Geometry: final body of the model. Coordinates: model frame, mm. A direction names the side the tool comes from. Give positions to 0.01 mm unless a question says otherwise; leave off trailing zeros. Order: outer loops, then holes, each group sorted by start corner. A loop starts at its lowest first (then second) coordinate and runs counter-clockwise, first axis right, second up. Notation, with made-up numbers: (-15, 27) - (38, 27) arc R20 cw to (38, 54) - close; hole circle Ø4 at (18.5, 75.25). An arc over 180 degrees is marked (long way). Use one line per item in the form item = value.
from build123d import *

# Parameters (mm, degrees)
SKETCH1_R           = 1.5
BOSS_EXTRUDE1_DEPTH = 1.5


with BuildPart() as part:
    # Sketch1 → Boss-Extrude1 (new body)
    with BuildSketch(Plane(origin=(0, 0, 0), x_dir=(1, 0, 0), z_dir=(0, 1, 0))):
        with BuildLine():
            Line((6.755042478, -2), (69.244957522, -2))
            ThreePointArc((69.244957522, -2), (70.169022091, -2.617763592), (69.951379765, -3.707790657))
            Line((69.951379765, -3.707790657), (67.996333944, -5.65905667))
            ThreePointArc((67.996333944, -5.65905667), (67.993254266, -9.902722426), (72.236921016, -9.903748986))
            Line((72.236921016, -9.903748986), (74.292893219, -7.847776783))
            ThreePointArc((74.292893219, -7.847776783), (75.382683432, -7.631004031), (76, -8.554883564))
            Line((76, -8.554883564), (76, -49.445116436))
            ThreePointArc((76, -49.445116436), (75.382683432, -50.368995969), (74.292893219, -50.152223217))
            Line((74.292893219, -50.152223217), (72.236921016, -48.096251014))
            ThreePointArc((72.236921016, -48.096251014), (67.993254266, -48.097277574), (67.996333944, -52.34094333))
            Line((67.996333944, -52.34094333), (69.951379765, -54.292209343))
            ThreePointArc((69.951379765, -54.292209343), (70.169022091, -55.382236408), (69.244957522, -56))
            Line((69.244957522, -56), (6.755042478, -56))
            ThreePointArc((6.755042478, -56), (5.830977909, -55.382236408), (6.048620235, -54.292209343))
            Line((6.048620235, -54.292209343), (8.003666056, -52.34094333))
            ThreePointArc((8.003666056, -52.34094333), (8.006745734, -48.097277574), (3.763078984, -48.096251014))
            Line((3.763078984, -48.096251014), (1.707106781, -50.152223217))
            ThreePointArc((1.707106781, -50.152223217), (0.617316568, -50.368995969), (0, -49.445116436))
            Line((0, -49.445116436), (0, -8.554883564))
            ThreePointArc((0, -8.554883564), (0.617316568, -7.631004031), (1.707106781, -7.847776783))
            Line((1.707106781, -7.847776783), (3.763078984, -9.903748986))
            ThreePointArc((3.763078984, -9.903748986), (8.006745734, -9.902722426), (8.003666056, -5.65905667))
            Line((8.003666056, -5.65905667), (6.048620235, -3.707790657))
            ThreePointArc((6.048620235, -3.707790657), (5.830977909, -2.617763592), (6.755042478, -2))
        make_face()
        with Locations(Location((11.0125, -13.001163208, 0), (0, 0, 270))):
            Circle(SKETCH1_R, mode=Mode.SUBTRACT)
        with Locations(Location((64.9875, -13.001163208, 0), (0, 0, 90))):
            Circle(SKETCH1_R, mode=Mode.SUBTRACT)
        with Locations(Location((64.9875, -44.998836792, 0), (0, 0, 270))):
            Circle(SKETCH1_R, mode=Mode.SUBTRACT)
        with Locations(Location((11.0125, -44.998836792, 0), (0, 0, 90))):
            Circle(SKETCH1_R, mode=Mode.SUBTRACT)
    extrude(amount=BOSS_EXTRUDE1_DEPTH)


solid = part.part
(1) Reachability of faces 1 (the face through (68.96, 0.74, 53.3)), 2 (the face through (7.04, 0.74, 4.7)), 3 (the face through (2.72, 0.74, 8.86)), 4 (the face through (73.28, 0.74, 49.14)), 5 (the face through (38, 1, 2)) from +Z, -Z, +X, -X, +Y, -Y: full face, straight path, thin tool, end or side. Return the list, or none.
Computed values:
face_1 = +X, +Y, -Y
face_2 = -X, +Y, -Y
face_3 = -Z, +Y, -Y
face_4 = +Z, +Y, -Y
face_5 = -Z, +X, -X, +Y, -Y
(2) Ray query, line 1 along Z through (x, y) = (69, 1); line 2 along X through (y, z) = (1.45, 50); line 3 along X through (y, z) = (0.4, 7.5). Return the intervals inside material, ascending.
Computed values:
line_1 = 2 to 4.66, 10.57 to 47.43, 53.34 to 56
line_2 = 0.17 to 1.86, 8.88 to 67.12, 74.14 to 75.83
line_3 = 8.87 to 67.13
(3) Cut plane B-B on x = 5. Output: boundary loops of the cut face in (y, z).
Computed values:
outline = (0, 10.65) - (1.5, 10.65) - (1.5, 47.35) - (0, 47.35) - close
(4) Cut plane A-A on y = 0.55. Output: boundary loops of the cut face in (x, z), plus the area to 3 significant figures.
Computed values:
outline = (0, 8.55) arc R1 ccw to (1.71, 7.85) - (3.76, 9.9) arc R3 cw to (8, 5.66) - (6.05, 3.71) arc R1 ccw to (6.76, 2) - (69.24, 2) arc R1 ccw to (69.95, 3.71) - (68, 5.66) arc R3 cw to (72.24, 9.9) - (74.29, 7.85) arc R1 ccw to (76, 8.55) - (76, 49.45) arc R1 ccw to (74.29, 50.15) - (72.24, 48.1) arc R3 cw to (68, 52.34) - (69.95, 54.29) arc R1 ccw to (69.24, 56) - (6.76, 56) arc R1 ccw to (6.05, 54.29) - (8, 52.34) arc R3 cw to (3.76, 48.1) - (1.71, 50.15) arc R1 ccw to (0, 49.45) - close; hole circle Ø3 at (11.01, 13); hole circle Ø3 at (11.01, 45); hole circle Ø3 at (64.99, 13); hole circle Ø3 at (64.99, 45)
area = 3,850 mm²
(5) Pull-direction query (X, two-part tool) for faces 6 (the face through (0, 1, 29)), 7 (the face through (65.9, 0.74, 14.19)), 8 (the face through (70.175, 0.74, 55.367)), 9 (the face through (2.75, 0.74, 49.11)); classes: released by +X, released by -X, zero draft, split by the parting line, or undercut.
Computed values:
face_6 = released by -X
face_7 = undercut
face_8 = released by +X
face_9 = undercut
